Autodesk Inventor part; units mm, degrees
ref_plane "Work Plane1" through (0, 0, -27.5) normal (0, 0, 1) x (1, 0, 0)
ref_plane "Work Plane2" through (0, 0, 32.5) normal (0, 0, 1) x (1, 0, 0)
ref_plane "YZ Plane" through (0, 0, 0) normal (1, 0, 0) x (0, 1, 0)
sketch "Sketch1" plane through (0, 0, 0) normal (0, 0, 1) x (1, 0, 0)
  line L0 (25, 7) -> (-25, 7)
  line L1 (-25, 7) -> (-25, 0)
  line L2 (-25, 0) -> (25, 0)
  line L3 (25, 0) -> (25, 7)
  circle A0 centre (-19, 3.5) radius 1.6
  circle A1 centre (19, 3.5) radius 1.6
  line L4 (19, 3.5) -> (-19, 3.5) construction
  line L5 (19, 3.5) -> (25, 7) construction
  line L6 (19, 3.5) -> (25, 0) construction
  line L7 (-19, 3.5) -> (-25, 7) construction
  line L8 (-19, 3.5) -> (-25, 0) construction
  line L9 (0, 0) -> (-19, 3.5) construction
  line L10 (0, 0) -> (19, 3.5) construction
  dimension "d0" = 3.2
  dimension "d1" = 38
  dimension "d2" = 7
  dimension "d3" = 50
extrude "Extrusion1" add sketch "Sketch1" along normal blind 5
sketch "Sketch2" plane through (-25, 7, 0) normal (0, 1, 0) x (1, 0, 0)
  line L0 (2.25, -3.5) -> (10, -3.5)
  line L1 (47.75, -3.5) -> (47.75, -1.5)
  line L2 (47.75, -1.5) -> (40, -1.5)
  line L3 (2.25, -1.5) -> (2.25, -3.5)
  line L4 (50, -5) -> (0, -5) construction
  line L5 (0, -5) -> (2.25, -3.5) construction
  line L6 (50, 0) -> (0, 0) construction
  line L7 (2.25, -1.5) -> (0, 0) construction
  line L8 (50, 0) -> (50, -5) construction
  line L9 (47.75, -3.5) -> (50, -5) construction
  line L10 (40, -3.5) -> (40, -5)
  line L11 (40, -5) -> (10, -5)
  line L12 (10, -5) -> (10, -3.5)
  line L13 (10, -1.5) -> (10, 0)
  line L14 (10, 0) -> (40, 0)
  line L15 (40, 0) -> (40, -1.5)
  line L16 (40, -3.5) -> (47.75, -3.5)
  line L17 (40, -1.5) -> (10, -1.5) construction
  line L18 (10, -3.5) -> (40, -3.5) construction
  line L19 (10, -1.5) -> (2.25, -1.5)
  line L20 (47.75, -3.5) -> (40, -5) construction
  line L21 (40, 0) -> (47.75, -1.5) construction
  line L22 (10, -5) -> (2.25, -3.5) construction
  line L23 (2.25, -1.5) -> (10, 0) construction
  point P0 (25, 0)
  dimension "d6" = 45.5
  dimension "d7" = 2
  dimension "d13" = 30
extrude "Extrusion2" cut sketch "Sketch2" against normal up to next
sketch "Sketch3" plane through (-25, 0, 0) normal (0, -1, 0) x (1, 0, 0)
  circle A0 centre (25, 2.5) radius 30
  line L0 (0, 5) -> (50, 5) construction
  line L1 (0, 5) -> (25, 2.5) construction
  line L2 (0, 0) -> (50, 0) construction
  line L3 (25, 2.5) -> (0, 0) construction
  line L4 (25, 2.5) -> (50, 5) construction
  point P0 (25, 0)
  dimension "d10" = 60
extrude "Extrusion3" add sketch "Sketch3" along normal blind 21
ref_plane "Work Plane1" through (0, 0, -27.5) normal (0, 0, 1) x (1, 0, 0)
sketch "Sketch5" plane through (0, 0, -27.5) normal (0, 0, 1) x (1, 0, 0)
  line L0 (14, -1.5) -> (-14, -1.5)
  line L1 (-14, -1.5) -> (-14, -19.5)
  line L2 (-14, -19.5) -> (14, -19.5)
  line L3 (14, -19.5) -> (14, -1.5)
  line L4 (-30, -21) -> (30, -21) construction
  line L5 (30, 0) -> (-30, 0) construction
  line L6 (30, 0) -> (-30, 0) construction
  line L7 (30, 0) -> (14, -1.5) construction
  line L8 (-14, -1.5) -> (-30, 0) construction
  line L9 (-30, -21) -> (30, -21) construction
  line L10 (-30, -21) -> (-14, -19.5) construction
  point P0 (0, 0)
  dimension "d16" = 18
  dimension "d17" = 28
extrude "Extrusion4" cut sketch "Sketch5" along normal blind 50
fillet "Fillet1" radius 3 8 edges at (15, 7, 0.75) (15, 7, 4.25) (15, 0, 4.25) (15, 0, 0.75) (-15, 0, 0.75) (-15, 7, 0.75) (-15, 7, 4.25) (-15, 0, 4.25)
fillet "Fillet2" radius 2 1 edges at (-30, 0, 2.5)
sketch "Sketch7" plane through (0, 0, 32.5) normal (0, 0, 1) x (1, 0, 0)
  spline S0 degree 3 poles (3.6755, -17.8887) (1.3417, -19.2361) (-1.5336, -19.2361) (-3.8674, -17.8887) knots 0 0 0 0 1 1 1 1
  line L0 (3.6755, -17.8887) -> (1.3417, -19.2361) construction
  line L1 (1.3417, -19.2361) -> (-1.5336, -19.2361) construction
  line L2 (-1.5336, -19.2361) -> (-3.8674, -17.8887) construction
  spline S1 degree 3 poles (-3.8674, -17.8887) (-6.2011, -16.5413) (-7.6388, -14.0512) (-7.6388, -11.3564) knots 0 0 0 0 1 1 1 1
  line L3 (-3.8674, -17.8887) -> (-6.2011, -16.5413) construction
  line L4 (-6.2011, -16.5413) -> (-7.6388, -14.0512) construction
  line L5 (-7.6388, -14.0512) -> (-7.6388, -11.3564) construction
  spline S2 degree 3 poles (-7.6388, -11.3564) (-7.6388, -8.6616) (-6.2011, -6.1715) (-3.8674, -4.8241) knots 0 0 0 0 1 1 1 1
  line L6 (-7.6388, -11.3564) -> (-7.6388, -8.6616) construction
  line L7 (-7.6388, -8.6616) -> (-6.2011, -6.1715) construction
  line L8 (-6.2011, -6.1715) -> (-3.8674, -4.8241) construction
  spline S3 degree 3 poles (-3.8674, -4.8241) (-1.5336, -3.4767) (1.3417, -3.4767) (3.6755, -4.8241) knots 0 0 0 0 1 1 1 1
  line L9 (-3.8674, -4.8241) -> (-1.5336, -3.4767) construction
  line L10 (-1.5336, -3.4767) -> (1.3417, -3.4767) construction
  line L11 (1.3417, -3.4767) -> (3.6755, -4.8241) construction
  spline S4 degree 3 poles (3.6755, -4.8241) (6.0092, -6.1715) (7.4469, -8.6616) (7.4469, -11.3564) knots 0 0 0 0 1 1 1 1
  line L12 (3.6755, -4.8241) -> (6.0092, -6.1715) construction
  line L13 (6.0092, -6.1715) -> (7.4469, -8.6616) construction
  line L14 (7.4469, -8.6616) -> (7.4469, -11.3564) construction
  spline S5 degree 3 poles (7.4469, -11.3564) (7.4469, -14.0512) (6.0092, -16.5413) (3.6755, -17.8887) knots 0 0 0 0 1 1 1 1
  line L15 (7.4469, -11.3564) -> (7.4469, -14.0512) construction
  line L16 (7.4469, -14.0512) -> (6.0092, -16.5413) construction
  line L17 (6.0092, -16.5413) -> (3.6755, -17.8887) construction
  spline S6 degree 3 poles (-0.623, -14.5187) (-0.623, -14.5201) (-0.623, -15.9241) (-2.0285, -15.9241) knots 0 0 0 0 1 1 1 1
  line L18 (-0.623, -14.5187) -> (-0.623, -14.5187) construction
  line L19 (-0.623, -14.5187) -> (-0.623, -15.9241) construction
  line L20 (-0.623, -15.9241) -> (-2.0285, -15.9241) construction
  spline S7 degree 3 poles (-2.0285, -15.9241) (-3.4339, -15.9241) (-3.4339, -14.5201) (-3.4339, -14.5187) knots 0 0 0 0 1 1 1 1
  line L21 (-2.0285, -15.9241) -> (-3.4339, -15.9241) construction
  line L22 (-3.4339, -15.9241) -> (-3.4339, -14.5187) construction
  line L23 (-3.4339, -14.5187) -> (-3.4339, -14.5187) construction
  line L24 (-0.623, -5.7345) -> (-0.623, -14.5187)
  spline S8 degree 3 poles (-4.488, -14.5187) (-4.488, -14.5211) (-4.488, -16.9782) (-2.0285, -16.9782) knots 0 0 0 0 1 1 1 1
  line L25 (-4.488, -14.5187) -> (-4.488, -14.5187) construction
  line L26 (-4.488, -14.5187) -> (-4.488, -16.9782) construction
  line L27 (-4.488, -16.9782) -> (-2.0285, -16.9782) construction
  spline S9 degree 3 poles (-2.0285, -16.9782) (0.4311, -16.9782) (0.4311, -14.5211) (0.4311, -14.5187) knots 0 0 0 0 1 1 1 1
  line L28 (-2.0285, -16.9782) -> (0.4311, -16.9782) construction
  line L29 (0.4311, -16.9782) -> (0.4311, -14.5187) construction
  line L30 (0.4311, -14.5187) -> (0.4311, -14.5187) construction
  line L31 (-3.4339, -14.5187) -> (-4.488, -14.5187)
  spline S10 degree 3 poles (1.8366, -14.5187) (1.839, -14.5187) (4.2961, -14.5187) (4.2961, -12.0591) knots 0 0 0 0 1 1 1 1
  line L32 (1.8366, -14.5187) -> (1.8366, -14.5187) construction
  line L33 (1.8366, -14.5187) -> (4.2961, -14.5187) construction
  line L34 (4.2961, -14.5187) -> (4.2961, -12.0591) construction
  spline S11 degree 3 poles (4.2961, -12.0591) (4.2961, -11.0712) (3.8992, -10.4803) (3.4243, -10.1266) knots 0 0 0 0 1 1 1 1
  line L35 (4.2961, -12.0591) -> (4.2961, -11.0712) construction
  line L36 (4.2961, -11.0712) -> (3.8992, -10.4803) construction
  line L37 (3.8992, -10.4803) -> (3.4243, -10.1266) construction
  spline S12 degree 3 poles (3.4243, -10.1266) (3.8992, -9.7729) (4.2961, -9.182) (4.2961, -8.1941) knots 0 0 0 0 1 1 1 1
  line L38 (3.4243, -10.1266) -> (3.8992, -9.7729) construction
  line L39 (3.8992, -9.7729) -> (4.2961, -9.182) construction
  line L40 (4.2961, -9.182) -> (4.2961, -8.1941) construction
  spline S13 degree 3 poles (4.2961, -8.1941) (4.2961, -5.7345) (1.839, -5.7345) (1.8366, -5.7345) knots 0 0 0 0 1 1 1 1
  line L41 (4.2961, -8.1941) -> (4.2961, -5.7345) construction
  line L42 (4.2961, -5.7345) -> (1.8366, -5.7345) construction
  line L43 (1.8366, -5.7345) -> (1.8366, -5.7345) construction
  line L44 (0.4311, -14.5187) -> (1.8366, -14.5187)
  line L45 (1.8366, -5.7345) -> (-0.623, -5.7345)
  spline S14 degree 3 poles (1.8366, -6.7886) (1.838, -6.7886) (3.242, -6.7886) (3.242, -8.1941) knots 0 0 0 0 1 1 1 1
  line L46 (1.8366, -6.7886) -> (1.8366, -6.7886) construction
  line L47 (1.8366, -6.7886) -> (3.242, -6.7886) construction
  line L48 (3.242, -6.7886) -> (3.242, -8.1941) construction
  spline S15 degree 3 poles (3.242, -8.1941) (3.242, -9.5995) (1.838, -9.5995) (1.8366, -9.5995) knots 0 0 0 0 1 1 1 1
  line L49 (3.242, -8.1941) -> (3.242, -9.5995) construction
  line L50 (3.242, -9.5995) -> (1.8366, -9.5995) construction
  line L51 (1.8366, -9.5995) -> (1.8366, -9.5995) construction
  line L52 (0.4311, -6.7886) -> (1.8366, -6.7886)
  line L53 (1.8366, -9.5995) -> (0.4311, -9.5995)
  line L54 (0.4311, -9.5995) -> (0.4311, -6.7886)
  spline S16 degree 3 poles (1.8366, -10.6536) (1.838, -10.6536) (3.242, -10.6536) (3.242, -12.0591) knots 0 0 0 0 1 1 1 1
  line L55 (1.8366, -10.6536) -> (1.8366, -10.6536) construction
  line L56 (1.8366, -10.6536) -> (3.242, -10.6536) construction
  line L57 (3.242, -10.6536) -> (3.242, -12.0591) construction
  spline S17 degree 3 poles (3.242, -12.0591) (3.242, -13.4646) (1.838, -13.4646) (1.8366, -13.4646) knots 0 0 0 0 1 1 1 1
  line L58 (3.242, -12.0591) -> (3.242, -13.4646) construction
  line L59 (3.242, -13.4646) -> (1.8366, -13.4646) construction
  line L60 (1.8366, -13.4646) -> (1.8366, -13.4646) construction
  line L61 (0.4311, -10.6536) -> (1.8366, -10.6536)
  line L62 (1.8366, -13.4646) -> (0.4311, -13.4646)
  line L63 (0.4311, -13.4646) -> (0.4311, -10.6536)
  point P0 (0, 0)
properties part number "Base with 9V Batt"
The listing builds one solid part. Answer for the finished solid, in the listing's coordinates (mm). A direction names the side the tool comes from. Give positions to 0.01 mm unless a question says otherwise; leave off trailing zeros. Write each loop counter-clockwise with the first axis right and the second up, starting at its lowest first coordinate (ties: lowest second). Pieces come first, ordered by that corner, then holes. Notation, with made-up numbers: (59.25, 0) - (67.25, 0) arc R17 ccw to (67.25, 4) - close; hole circle Ø3 at (-15, 4.25). An arc over 180 degrees is marked (long way). Use a Markdown table: item, result.
1. Each of these flat-tipped pins is pushed along its axis until it touches: P1, Ø1, axis at y = 2, z = 2, coming from the -X side; P2, Ø3.5, axis at x = -18, y = 4, coming from the -Z side; P3, Ø4, axis at y = 4.5, z = 3.5, coming from the +X side. Where does it stop, or does it pass through?
Values follow:
| item | result |
|---|---|
| P1 | stops at x = -25 |
| P2 | stops at z = 0 |
| P3 | stops at x = 25 |
2. A tool of negligible diameter and unlimited length cuts with its end or side. For faces 1 (the flat face through (-22.75, 4, 2)), 2 (the flat face through (14, -11, -1)), 3 (the cylindrical face through (14.14, 0.9, 4.24)), from which of +Z, -Z, +X, -X, +Y, -Y can it reach the whole face along a straight path? Write none if from no direction.
Values follow:
| item | result |
|---|---|
| face 1 | +Y |
| face 2 | -Z |
| face 3 | +Z, -Z, +Y |
3. Section C-C on x = -19 is taken. Count the separate pieces of the cut face and the enclosed holes in it, plus the area to 3 significant figures.
Values follow:
| item | result |
|---|---|
| separate pieces | 3 |
| enclosed holes | 0 |
| area | 984 mm² |
4. Section B-B on y = -11 is taken. Write down the section's boundary in (x, z).
Values follow:
| item | result |
|---|---|
| outline | (-14, -24.03) - (-14, 22.5) - (14, 22.5) - (14, -24.03) arc R30 ccw (long way) to start |
5. Section A-A on x = 0 is taken. Write down the section's boundary in (y, z).
Values follow:
| item | result |
|---|---|
| outline | (-21, -27.5) - (-19.5, -27.5) - (-19.5, 22.5) - (-1.5, 22.5) - (-1.5, -27.44) arc R2 ccw to (0, -25.5) - (0, 30.5) arc R2 ccw to (-2, 32.5) - (-21, 32.5) - close |
6. Find the intervals of material crossed by probe 1 along X at (y, z) = (3.5, 3.9); probe 2 along Y at (x, z) = (-5, -1); probe 3 along Z at (x, y) = (20, 5), in increasing order. Write a range as from..to.
Values follow:
| item | result |
|---|---|
| probe 1 | x = -25..-20.6, -17.4..-15, 15..17.4, 20.6..25 |
| probe 2 | y = -21..-19.5, -1.5..0 |
| probe 3 | z = 0..1.5, 3.5..5 |
7. For a pull along Y with two mould halves and no side action, classify faces 4 (the flat face through (21, 4, 0)), 5 (the cylindrical face through (-20.18, 2.42, 0.74)), 6 (the cylindrical face through (14.14, 0.9, 0.74)) as released by +Y, released by -Y, zero draft, split by the parting line, or undercut.
Values follow:
| item | result |
|---|---|
| face 4 | zero draft |
| face 5 | undercut |
| face 6 | released by +Y |
